Part model, mm, in its own coordinate system. Face numbers are marked on the shaded views. A direction names the side the tool comes from. Coordinates: 2 decimals unless noted, no trailing zeros. Loops run counter-clockwise (first coordinate to the right, second up) from the corner with the lowest first, then second, coordinate; pieces in that order, holes last. Notation, with made-up numbers: (17.25, 75.5) -> (52.25, 75.5) arc R19 ccw to (52.25, 87.5) -> close; hole circle Ø10 at (43, -5). An arc over 180 degrees is marked (long way). Use one line per item in the form item = value. Start each with the question number.
(1) Band-saw the part on A-A on y = -35.25. Give the cut face in (x, z).
(2) Band-saw the part on D-D on y = -11. Give the cut face in (x, z), then the cut area to 3 significant figures.
(3) Pin check, flat tips, straight feed: P1, Ø13, axis at x = 19.5, y = -17.5, coming from the +Z side; P2, Ø5, axis at y = -35.25, z = -70, coming from the +X side; P3, Ø8, axis at x = 17.5, y = -30, coming from the -Z side; P4, Ø3.5, axis at y = 30.25, z = -70, coming from the -X side. Stop position of each tip, or through.
(4) Band-saw the part on C-C on x = 22. Give the cut face in (y, z), then the cut area to 3 significant figures.
(5) Band-saw the part on B-B on z = -70. Give the cut face in (x, y), then the cut area to 3 significant figures.
(6) Drill centre lines: L1, parallel to Y at x = 3, z = -70; L2, parallel to Z at x = 12, y = 10; L3, parallel to Z at x = 2, y = 30. Where is each one in solid material? Low to high. Write a range as [from, to].
(7) 3-axis set-ups, long thin cutter, end or side, ignore diameter. For the marked faces 1, 2 and 3: which of +Z, -Z, +X, -X, +Y, -Y reach the whole face in a straight line?
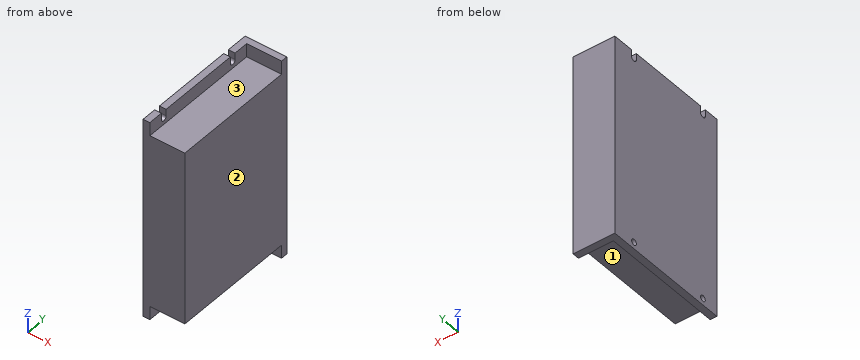
```python
from build123d import *

# Parameters (mm, degrees)
SKETCH_1_W          = 150
SKETCH_1_H          = 97
EXTRUDE_1_DEPTH     = 31
SKETCH_2_W          = 10
SKETCH_2_H          = 92
CUT_EXTRUDE_1_DEPTH = 26
SKETCH_3_R          = 2.25
CUT_EXTRUDE_2_DEPTH = 26


with BuildPart() as part:
    # 草图1 → 凸台-拉伸1 (new body)
    with BuildSketch(Plane(origin=(0, 0, 0), x_dir=(0, 0, -1), z_dir=(1, 0, 0))):
        Rectangle(SKETCH_1_W, SKETCH_1_H)
    extrude(amount=EXTRUDE_1_DEPTH)

    # 草图2 → 切除-拉伸1 (cut)
    with BuildSketch(Plane(origin=(31, 0, 0), x_dir=(0, 0, -1), z_dir=(1, 0, 0))):
        with Locations((-70, -2.5)):
            Rectangle(SKETCH_2_W, SKETCH_2_H)
        with Locations((70, -2.5)):
            Rectangle(SKETCH_2_W, SKETCH_2_H)
    extrude(amount=-CUT_EXTRUDE_1_DEPTH, mode=Mode.SUBTRACT)

    # 草图3 → 切除-拉伸2 (cut)
    with BuildSketch(Plane(origin=(5, 0, 0), x_dir=(0, 0, -1), z_dir=(1, 0, 0))):
        with Locations((70, 30.25)):
            Circle(SKETCH_3_R)
        with Locations((70, -35.25)):
            Circle(SKETCH_3_R)
        with BuildLine():
            Line((-70, 32.5), (-75, 32.5))
            Line((-75, 32.5), (-75, 28))
            Line((-75, 28), (-70, 28))
            ThreePointArc((-70, 28), (-67.75, 30.25), (-70, 32.5))
        make_face()
        with BuildLine():
            Line((-70, -33), (-75, -33))
            Line((-75, -33), (-75, -37.5))
            Line((-75, -37.5), (-70, -37.5))
            ThreePointArc((-70, -37.5), (-67.75, -35.25), (-70, -33))
        make_face()
    extrude(amount=-CUT_EXTRUDE_2_DEPTH, mode=Mode.SUBTRACT)


solid = part.part
```
A:
q1.outline = (0, -75) -> (5, -75) -> (5, -72.25) -> (0, -72.25) -> close; (0, -67.75) -> (5, -67.75) -> (5, -65) -> (31, -65) -> (31, 65) -> (5, 65) -> (5, 67.75) -> (0, 67.75) -> close
q2.outline = (0, -75) -> (5, -75) -> (5, -65) -> (31, -65) -> (31, 65) -> (5, 65) -> (5, 75) -> (0, 75) -> close
q2.area = 4,130 mm²
q3.P1 = 65
q3.P2 = 5
q3.P3 = -65
q3.P4 = through
q4.outline = (-48.5, -65) -> (43.5, -65) -> (43.5, -75) -> (48.5, -75) -> (48.5, 75) -> (43.5, 75) -> (43.5, 65) -> (-48.5, 65) -> close
q4.area = 12,700 mm²
q5.outline = (0, -48.5) -> (5, -48.5) -> (5, -37.5) -> (0, -37.5) -> close; (0, -33) -> (5, -33) -> (5, 28) -> (0, 28) -> close; (0, 32.5) -> (5, 32.5) -> (5, 43.5) -> (31, 43.5) -> (31, 48.5) -> (0, 48.5) -> close
q5.area = 570 mm²
q6.L1 = [-48.5, -37.5], [-33, 28], [32.5, 48.5]
q6.L2 = [-65, 65]
q6.L3 = [-75, -72.24], [-67.76, 67.76]
q7.face_1 = -Z, +X, -Y
q7.face_2 = +Z, -Z, +X, +Y, -Y
q7.face_3 = +Z, +X, -Y
